from build123d import *

# Parameters (mm, degrees)
SKETCH16_R                 = 3.4
SKETCH16_R_2               = 6
BOSS_EXTRUDE3_DEPTH        = 10
F_3_5_3_5_DIAMETER_HOLE1_D = 3.5


with BuildPart() as part:
    # Sketch16 → Boss-Extrude3 (new body)
    with BuildSketch(Plane.XY):
        with BuildLine():
            Line((-35, 10), (35, 10))
            ThreePointArc((35, 10), (45, 0), (35, -10))
            Line((35, -10), (-35, -10))
            ThreePointArc((-35, -10), (-45, 0), (-35, 10))
        make_face()
        with Locations((-35.355, 0)):
            Circle(SKETCH16_R, mode=Mode.SUBTRACT)
        Circle(SKETCH16_R_2, mode=Mode.SUBTRACT)
        with Locations(Location((35.355, 0, 0), (0, 0, 180))):
            Circle(SKETCH16_R, mode=Mode.SUBTRACT)
    extrude(amount=BOSS_EXTRUDE3_DEPTH)

    # Ø3.5 (3.5) Diameter Hole1 (through all)
    with Locations(Plane(origin=(0, 10, 0), x_dir=(1, 0, 0), z_dir=(0, 1, 0))):
        with Locations((0, -5)):
            Hole(F_3_5_3_5_DIAMETER_HOLE1_D / 2)


solid = part.part
Input: part model. Units: mm. Frame: model coordinates. Round coordinates to 2 decimals unless told otherwise and drop trailing zeros. Loops run counter-clockwise (first coordinate to the right, second up) from the corner with the lowest first, then second, coordinate; pieces in that order, holes last. Notation, with made-up numbers: M 28.25,-19.75 L 69.25,-19.75 A24 cw 69.25,1.25 Z; hole C -4,61.25 d7. An arc over 180 degrees is marked long. Answer as CSV lines item,"result". Start each with the question number.
(1) Draft query along Z for faces 1 (the cylindrical face through (-38.75, 0.15, 4.93)), 2 (the cylindrical face through (0.38, -7.9, 6.71)), 3 (the flat face through (1, -7, 0)), 4 (the flat face through (1, -7, 10)). Return one class per face: released by +Z, released by -Z, zero draft, split by the parting line, or undercut.
(2) Section C-C, the plane y = 0. Output: boundary loops of the cut face in (x, z) (3 decimals).
(3) First-contact query: pin 1 (3 mm diameter, centred on x = 0, z = 5, fed in from -Y); pin 2 (2 mm diameter, centred on y = -1.5, z = 5, fed in from +X); pin 3 (6 mm diameter, centred on y = -7, z = 8, fed in from -X). Flat tips, straight axial feed; report the tip coordinate or a pass-through.
(4) Section D-D, the plane z = 1.25. Output: boundary loops of the cut face in (x, y) (3 decimals).
(5) Section B-B, the plane x = 0. Output: boundary loops of the cut face in (y, z).
(6) Section A-A, the plane z = 5. Output: boundary loops of the cut face in (x, y) (3 decimals), plus the area to 3 significant figures.
(7) Line query: line 1 (X direction, y = -0.5, z = 3.5); line 2 (Y direction, x = 0, z = 2.25); line 3 (X direction, y = -2, z = 7). Output: solid intervals per line, ascending. Write a range as [from, to].
Values found:
1,face 1,"zero draft"
1,face 2,"undercut"
1,face 3,"released by -Z"
1,face 4,"released by +Z"
2,outline,"M -45,0 L -38.755,0 L -38.755,10 L -45,10 Z; M -31.955,0 L -6,0 L -6,10 L -31.955,10 Z; M 6,0 L 31.955,0 L 31.955,10 L 6,10 Z; M 38.755,0 L 45,0 L 45,10 L 38.755,10 Z"
3,pin 1,"passes through"
3,pin 2,"stops at x = 44.99"
3,pin 3,"stops at x = -44.17"
4,outline,"M -35,-10 L 35,-10 A10 ccw 35,10 L -35,10 A10 ccw Z; hole C -35.355,0 d6.8; hole C 0,0 d12; hole C 35.355,0 d6.8"
5,outline,"M -10,0 L -6,0 L -6,3.25 L -10,3.25 Z; M -10,6.75 L -6,6.75 L -6,10 L -10,10 Z; M 6,0 L 10,0 L 10,3.25 L 6,3.25 Z; M 6,6.75 L 10,6.75 L 10,10 L 6,10 Z"
6,outline,"M -35,-10 L -1.75,-10 L -1.75,-5.739 A6 cw -1.75,5.739 L -1.75,10 L -35,10 A10 ccw Z; M 1.75,-10 L 35,-10 A10 ccw 35,10 L 1.75,10 L 1.75,5.739 A6 cw 1.75,-5.739 Z; hole C -35.355,0 d6.8; hole C 35.355,0 d6.8"
6,area,"1,500 mm²"
7,line 1,"x = [-44.99, -38.72], [-31.99, -5.98], [5.98, 31.99], [38.72, 44.99]"
7,line 2,"y = [-10, -6], [6, 10]"
7,line 3,"x = [-44.8, -38.1], [-32.61, -5.66], [5.66, 32.61], [38.1, 44.8]"
